Read the model definition and answer for the solid it produces. Units are mm, in the model's axes. A direction names the side the tool comes from. Round coordinates to 2 decimals unless told otherwise and drop trailing zeros. Loops run counter-clockwise (first coordinate to the right, second up) from the corner with the lowest first, then second, coordinate; pieces in that order, holes last. Notation, with made-up numbers: (9, 84.25) -> (51, 84.25) arc R28 ccw to (51, 109.25) -> close; hole circle Ø5 at (21.5, 6). An arc over 180 degrees is marked (long way). Put each result on its own line as item: value.
from build123d import *

# Parameters (mm, degrees)
IZIM1_W                          = 23
IZIM1_H                          = 15.5
Y_KSEKLIK_EKSTR_ZYON1_DEPTH      = 24.5
IZIM2_W                          = 21.4
IZIM2_H                          = 7
IZIM2_W_2                        = 5
IZIM2_H_2                        = 6
IZIM2_W_3                        = 4
IZIM2_H_3                        = 7.5
KES_EKSTR_ZYON1_DEPTH            = 24.5
IZIM3_R                          = 0.75
Y_KSEKLIK_EKSTR_ZYON4_DEPTH      = 2.5
Y_KSEKLIK_EKSTR_ZYON4_DEPTH_BACK = 10
IZIM8_R                          = 1.5
KES_EKSTR_ZYON3_DEPTH            = 10


with BuildPart() as part:
    # Çizim1 → Yükseklik-Ekstrüzyon1 (new body)
    with BuildSketch(Plane(origin=(0, 0, 0), x_dir=(1, 0, 0), z_dir=(0, 1, 0))):
        Rectangle(IZIM1_W, IZIM1_H)
    extrude(amount=Y_KSEKLIK_EKSTR_ZYON1_DEPTH)

    # Çizim2 → Kes-Ekstrüzyon1 (cut)
    with BuildSketch(Plane(origin=(0, 0, 0), x_dir=(1, 0, 0), z_dir=(0, 1, 0))):
        with Locations((0, -4.25)):
            Rectangle(IZIM2_W, IZIM2_H)
        Polygon((-8.5, 1.153663729), (-7.5, 1.153663729), (-7.5, 7.75), (-10.5, 7.75), (-10.5, 1.153663729), (-9.5, 1.153663729), (-9.5, 0.25), (-8.5, 0.25), align=None)
        with Locations((0, 4.75)):
            Rectangle(IZIM2_W_2, IZIM2_H_2)
        with Locations((-5, 4)):
            Rectangle(IZIM2_W_3, IZIM2_H_3)
        with Locations((5, 4)):
            Rectangle(IZIM2_W_3, IZIM2_H_3)
        Polygon((10.5, 7.75), (7.5, 7.75), (7.5, 1.153663729), (8.5, 1.153663729), (8.5, 0.25), (9.5, 0.25), (9.5, 1.153663729), (10.5, 1.153663729), align=None)
    extrude(amount=KES_EKSTR_ZYON1_DEPTH, mode=Mode.SUBTRACT)

    # Çizim3 → Yükseklik-Ekstrüzyon4 (add, two sides)
    with BuildSketch(Plane(origin=(0, 24.5, 0), x_dir=(1, 0, 0), z_dir=(0, 1, 0))) as y_kseklik_ekstr_zyon4_sk:
        with Locations((-9, 0.701831864)):
            Circle(IZIM3_R)
        with Locations((9, 0.701831864)):
            Circle(IZIM3_R)
    extrude(amount=Y_KSEKLIK_EKSTR_ZYON4_DEPTH)
    extrude(y_kseklik_ekstr_zyon4_sk.sketch, amount=-Y_KSEKLIK_EKSTR_ZYON4_DEPTH_BACK)

    # Çizim5 → Döndür2 (revolve)
    with BuildSketch(Plane.ZY.offset(9)):
        with BuildLine():
            Line((-2.701831864, 26), (-0.701831864, 26))
            Line((-0.701831864, 26), (-0.701831864, 27))
            add(Edge.make_bspline(
                [(-2.701831864, 26), (-1.790219679, 26.874416791), (-0.701831864, 27)],
                knots=[0, 0, 0, 0.748833581, 0.748833581, 0.748833581], degree=2))
        make_face()
    revolve(axis=Axis((-9, 26, -0.701831864), (0, 1, 0)))

    # Çizim6 → Döndür3 (revolve)
    with BuildSketch(Plane(origin=(9, 0, 0), x_dir=(0, 0, -1), z_dir=(1, 0, 0))):
        with BuildLine():
            Line((-1.298168136, 26), (0.701831864, 26.01043139))
            Line((0.701831864, 26.01043139), (0.701831864, 27))
            add(Edge.make_bspline(
                [(-1.298168136, 26), (-0.38655595, 26.874416791), (0.701831864, 27)],
                knots=[0, 0, 0, 0.748833581, 0.748833581, 0.748833581], degree=2))
        make_face()
    revolve(axis=Axis((9, 26.01043139, -0.701831864), (0, 1, 0)))

    # Çizim8 → Kes-Ekstrüzyon3 (cut)
    with BuildSketch(Plane.XY.offset(0.75)):
        with Locations((0, 5.5)):
            Circle(IZIM8_R)
    extrude(amount=-KES_EKSTR_ZYON3_DEPTH, mode=Mode.SUBTRACT)


solid = part.part
Item 1: Flat-ended cylindrical pins translate along their axes: pin 1 Ø0.8 at (x, y) = (-8, 9.5) entering from -Z; pin 2 Ø1.5 at (x, y) = (5.5, 15) entering from -Z; pin 3 Ø3 at (x, y) = (4.5, 17) entering from +Z. Find the tip coordinate at first contact, or state that the pin passes through.
Derived:
pin 1: stops at z = -1.15
pin 2: stops at z = -0.25
pin 3: stops at z = 0.75
Item 2: Find the intervals of material crossed by line 1 along X through (y, z) = (6.75, -6.25); line 2 along X through (y, z) = (8.5, 5.5); line 3 along Y through (x, z) = (0, -1), in increasing order.
Derived:
line 1: x = -11.5 to -10.5, -7.5 to -7, -3 to -2.5, 2.5 to 3, 7 to 7.5, 10.5 to 11.5
line 2: x = -11.5 to -10.7, 10.7 to 11.5
line 3: y = 0 to 4, 7 to 24.5
Item 3: The part is cut by section A-A (z = -4). Determine the outline of the cut face in (x, y), then the cut area to 3 significant figures.
Derived:
outline: (-11.5, 0) -> (-10.5, 0) -> (-10.5, 24.5) -> (-11.5, 24.5) -> close; (-7.5, 0) -> (-7, 0) -> (-7, 24.5) -> (-7.5, 24.5) -> close; (-3, 0) -> (-2.5, 0) -> (-2.5, 24.5) -> (-3, 24.5) -> close; (2.5, 0) -> (3, 0) -> (3, 24.5) -> (2.5, 24.5) -> close; (7, 0) -> (7.5, 0) -> (7.5, 24.5) -> (7, 24.5) -> close; (10.5, 0) -> (11.5, 0) -> (11.5, 24.5) -> (10.5, 24.5) -> close
area: 98.0 mm^2
Item 4: The part is cut by section C-C (y = 25). Determine the outline of the cut face in (x, z).
Derived:
outline: circle Ø1.5 at (-9, -0.7); circle Ø1.5 at (9, -0.7)
Item 5: For a pull along X with two mould halves and no side action, classify faces 1 (the flat face through (-10.5, 12, -4)), 2 (the flat face through (9, 27, -1)), 3 (the flat face through (0, 12, 0.75)) as pulls with the +X half, pulls with the -X half, needs draft (parallel to the pull), parting line crosses it, or undercut.
Derived:
face 1: undercut
face 2: needs draft
face 3: undercut
Item 6: Which of the six approach directions +Z, -Z, +X, -X, +Y, -Y give full straight-line access (tool end or side, diameter ignored) to faces 4 (the flat face through (3, 12, -4)), 5 (the flat face through (-9, 7, -0.25)), 6 (the flat face through (11, 12, 7.75))?
Derived:
face 4: -Z, +Y, -Y
face 5: -Z, -Y
face 6: +Z, +X, -X, +Y, -Y
Item 7: The part is cut by section D-D (x = 3.5). Determine the outline of the cut face in (y, z).
Derived:
outline: (0, -0.25) -> (24.5, -0.25) -> (24.5, 0.75) -> (0, 0.75) -> close
Item 8: The part is cut by section B-B (x = 0). Determine the outline of the cut face in (y, z).
Derived:
outline: (0, -1.75) -> (4, -1.75) -> (4, 0.75) -> (0, 0.75) -> close; (7, -1.75) -> (24.5, -1.75) -> (24.5, 0.75) -> (7, 0.75) -> close
